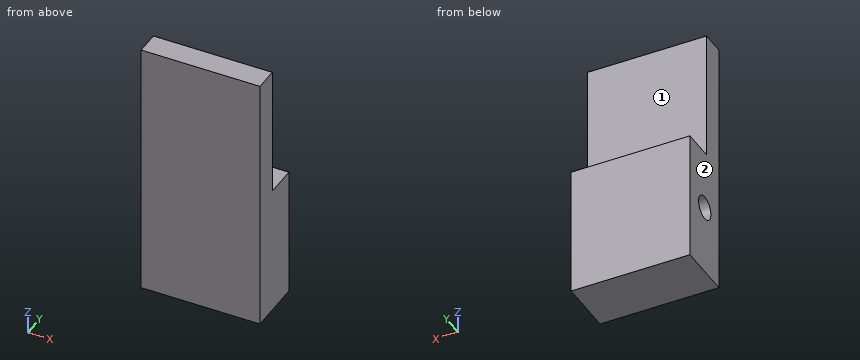
from build123d import *

# Parameters (mm, degrees)
SKETCH3_W           = 10
SKETCH3_H           = 22
BOSS_EXTRUDE1_DEPTH = 2
SKETCH4_W           = 10
SKETCH4_H           = 11
BOSS_EXTRUDE2_DEPTH = 2.7
SKETCH5_R           = 1
CUT_EXTRUDE1_DEPTH  = 2


with BuildPart() as part:
    # Sketch3 → Boss-Extrude1 (new body)
    with BuildSketch(Plane(origin=(0, 0, 0), x_dir=(1, 0, 0), z_dir=(0, 1, 0))):
        with Locations((-12.849765258, -8.469483568)):
            Rectangle(SKETCH3_W, SKETCH3_H)
    extrude(amount=BOSS_EXTRUDE1_DEPTH)

    # Sketch4 → Boss-Extrude2 (add)
    with BuildSketch(Plane(origin=(0, 2, 0), x_dir=(1, 0, 0), z_dir=(0, 1, 0))):
        with Locations((-12.849765258, -2.969483568)):
            Rectangle(SKETCH4_W, SKETCH4_H)
    extrude(amount=BOSS_EXTRUDE2_DEPTH)

    # Sketch5 → Cut-Extrude1 (cut)
    with BuildSketch(Plane.ZY.offset(17.849765258)):
        with Locations((3.369483568, 2.3)):
            Circle(SKETCH5_R)
    extrude(amount=-CUT_EXTRUDE1_DEPTH, mode=Mode.SUBTRACT)


solid = part.part
The listing builds one solid part. Answer for the finished solid, in the listing's coordinates (mm). Face numbers are marked on the shaded views. A direction names the side the tool comes from. Coordinates: 2 decimals unless noted, no trailing zeros. Write each loop counter-clockwise with the first axis right and the second up, starting at its lowest first coordinate (ties: lowest second). Pieces come first, ordered by that corner, then holes. Notation, with made-up numbers: (10.25, -29) - (57.25, -29) arc R28 cw to (57.25, 9) - close; hole circle Ø11 at (-8.75, -4.75). An arc over 180 degrees is marked (long way). Return JSON: item names as keys, results as strings.
1. Which of the six approach directions +Z, -Z, +X, -X, +Y, -Y give full straight-line access (tool end or side, diameter ignored) to the marked faces 1 and 2?
Final values:
{"face 1": "+Z, +X, -X, +Y", "face 2": "+Z, -Z, -X, +Y, -Y"}
2. The part is cut by section C-C on x = -12.25. Determine the outline of the cut face in (y, z).
Final values:
{"outline": "(0, -2.53) - (4.7, -2.53) - (4.7, 8.47) - (2, 8.47) - (2, 19.47) - (0, 19.47) - close"}
3. The part is cut by section D-D on z = 9. Determine the outline of the cut face in (x, y).
Final values:
{"outline": "(-17.85, 0) - (-7.85, 0) - (-7.85, 2) - (-17.85, 2) - close"}
4. Consider line 1 along Y through (x, z) = (-14.5, 10.5); line 2 along Z through (x, y) = (-9, 2.2); line 3 along Z through (x, y) = (-16.25, 2.6). Determine where each line is inside the solid, lowest interval first.
Final values:
{"line 1": "0 to 2", "line 2": "-2.53 to 8.47", "line 3": "-2.53 to 2.42, 4.32 to 8.47"}
5. Each of these flat-tipped pins is pushed along its axis until it touches: pin 1 Ø5 at (x, z) = (-13, 12.5) entering from +Y; pin 2 Ø0.8 at (x, y) = (-13.5, 3) entering from +Z; pin 3 Ø0.6 at (y, z) = (2.5, 3.5) entering from -X; pin 4 Ø6 at (x, z) = (-13, 10.5) entering from +Y. Where does it stop, or does it pass through?
Final values:
{"pin 1": "y = 2", "pin 2": "z = 8.47", "pin 3": "x = -15.85", "pin 4": "y = 4.7"}
6. The part is cut by section B-B on y = 2.3. Determine the outline of the cut face in (x, z), then the cut area to 3 significant figures.
Final values:
{"outline": "(-17.85, -2.53) - (-7.85, -2.53) - (-7.85, 8.47) - (-17.85, 8.47) - (-17.85, 4.37) - (-15.85, 4.37) - (-15.85, 2.37) - (-17.85, 2.37) - close", "area": "106 mm^2"}
7. The part is cut by section A-A on x = -16.25. Determine the outline of the cut face in (y, z).
Final values:
{"outline": "(0, -2.53) - (4.7, -2.53) - (4.7, 8.47) - (2, 8.47) - (2, 19.47) - (0, 19.47) - close; hole circle Ø2 at (2.3, 3.37)"}
